Work out the finished part from the listing and answer in its coordinate system (mm). A direction names the side the tool comes from. Coordinates: 2 decimals unless noted, no trailing zeros. Loops run counter-clockwise (first coordinate to the right, second up) from the corner with the lowest first, then second, coordinate; pieces in that order, holes last. Notation, with made-up numbers: M 23.5,43.25 L 49.5,43.25 A31 ccw 49.5,67.25 Z; hole C 69.5,-39.5 d7. An arc over 180 degrees is marked long. Write each question's results on one line, items separated by ' | '.
```python
from build123d import *

# Parameters (mm, degrees)
SKETCH1_W           = 40
SKETCH1_H           = 15
BOSS_EXTRUDE1_DEPTH = 15
CUT_EXTRUDE1_DEPTH  = 5
CUT_EXTRUDE2_DEPTH  = 13
FILLET3_R           = 2.5
FILLET4_R           = 2.5
SKETCH4_R           = 1.4
CUT_EXTRUDE3_DEPTH  = 8
SKETCH5_R           = 1
CUT_EXTRUDE4_DEPTH  = 10


with BuildPart() as part:
    # Sketch1 → Boss-Extrude1 (new body)
    with BuildSketch(Plane(origin=(0, 0, 0), x_dir=(1, 0, 0), z_dir=(0, 1, 0))):
        Rectangle(SKETCH1_W, SKETCH1_H)
    extrude(amount=BOSS_EXTRUDE1_DEPTH)

    # Sketch2 → Cut-Extrude1 (cut)
    with BuildSketch(Plane(origin=(20, 0, 0), x_dir=(0, 0, -1), z_dir=(1, 0, 0))):
        with BuildLine():
            Line((-2.5, 13.5), (-2.5, 7.5))
            Line((-2.5, 7.5), (2.5, 7.5))
            Line((2.5, 7.5), (2.5, 13.5))
            ThreePointArc((2.5, 13.5), (0, 16), (-2.5, 13.5))
        make_face()
    extrude(amount=-CUT_EXTRUDE1_DEPTH, mode=Mode.SUBTRACT)

    # Sketch3 → Cut-Extrude2 (cut)
    with BuildSketch(Plane(origin=(0, 15, 0), x_dir=(1, 0, 0), z_dir=(0, 1, 0))):
        Polygon((-18, 5.5), (-20, 5.5), (-20, -5.5), (-18, -5.5), (15, -5.5), (15, 2), (15, 5.5), align=None)
    extrude(amount=-CUT_EXTRUDE2_DEPTH, mode=Mode.SUBTRACT)

    # Fillet3
    fillet3_edges = [part.edges().sort_by_distance(p)[0] for p in [
        (17.5, 7.5, -2.5),
    ]]
    fillet(fillet3_edges, radius=FILLET3_R)

    # Fillet4
    fillet4_edges = [part.edges().sort_by_distance(p)[0] for p in [
        (17.5, 7.5, 2.5),
    ]]
    fillet(fillet4_edges, radius=FILLET4_R - 0.0001)  # a hair under: the kernel refuses the full size

    # Sketch4 → Cut-Extrude3 (cut)
    with BuildSketch(Plane(origin=(-14.629961684, 3.541693354, -7.5), x_dir=(-1, 0, 0), z_dir=(0, 0, -1))):
        with Locations((-6.629961684, 6.289794724)):
            Circle(SKETCH4_R)
    extrude(amount=-CUT_EXTRUDE3_DEPTH, mode=Mode.SUBTRACT)

    # Sketch5 → Cut-Extrude4 (cut)
    with BuildSketch(Plane(origin=(0, 2, 0), x_dir=(1, 0, 0), z_dir=(0, 1, 0))):
        with Locations(Location((-15.932700141, 0, 0), (0, 0, 270))):
            Circle(SKETCH5_R)
    extrude(amount=-CUT_EXTRUDE4_DEPTH, mode=Mode.SUBTRACT)


solid = part.part
```
1) For a pull along Z with two mould halves and no side action, classify faces 5 (the face through (0, 7, 7.5)), 6 (the face through (-3, 2, 0)), 7 (the face through (4, 15, 6)) as released by +Z, released by -Z, zero draft, split by the parting line, or undercut.
Check result:
face 5: released by +Z | face 6: undercut | face 7: zero draft
2) Given pin 1 Ø2 at (x, y) = (-8, 9.83) entering from -Z; pin 2 Ø3.5 at (x, z) = (-7, 0) entering from +Y; pin 3 Ø3.5 at (y, z) = (7, 0) entering from -X, each flat-ended and moving along its own axis, determine where each tip first touches the part or whether it passes through.
Check result:
pin 1: z = 5.5 | pin 2: y = 2 | pin 3: x = 15
3) Find section A-A, the plane x = -8. Give the vertices of the cut face in (y, z).
Check result:
outline: M 0,-7.5 L 8.43,-7.5 L 8.43,-5.5 L 2,-5.5 L 2,5.5 L 15,5.5 L 15,7.5 L 0,7.5 Z; M 11.23,-7.5 L 15,-7.5 L 15,-5.5 L 11.23,-5.5 Z
4) Which of the six approach directions +Z, -Z, +X, -X, +Y, -Y give full straight-line access (tool end or side, diameter ignored) to faces 1 (the face through (15, 7, 0)), 2 (the face through (17.54, 14.3, 2.37)), 3 (the face through (-6.6, 9.9, -6.5)), 4 (the face through (4, 15, -6))?
Check result:
face 1: -X, +Y | face 2: +X, -X | face 3: -Z | face 4: +Z, -Z, +X, -X, +Y
5) Find section D-D, the plane z = -3.5. Give the vertices of the cut face in (x, y), and give its area (3 significant figures).
Check result:
outline: M -20,0 L 20,0 L 20,15 L 15,15 L 15,2 L -20,2 Z | area: 145 mm^2
6) Find section B-B, the plane x = 11. Give the vertices of the cut face in (y, z).
Check result:
outline: M 0,-7.5 L 15,-7.5 L 15,-5.5 L 2,-5.5 L 2,5.5 L 15,5.5 L 15,7.5 L 0,7.5 Z
7) Find section C-C, the plane y = 2.75. Give the vertices of the cut face in (x, z).
Check result:
outline: M -20,-7.5 L 20,-7.5 L 20,7.5 L -20,7.5 L -20,5.5 L 15,5.5 L 15,-5.5 L -20,-5.5 Z
8) Straight lines are drawn through the part: probe 1 along Y at (x, z) = (-8, -6.05); probe 2 along X at (y, z) = (0.6, 0); probe 3 along Z at (x, y) = (-10, 2.5). For each, find the intervals that lie inside material, in ascending order. Write a range as [from, to].
Check result:
probe 1: [0, 8.43], [11.23, 15] | probe 2: [-20, -16.93], [-14.93, 20] | probe 3: [-7.5, -5.5], [5.5, 7.5]
